Can you work these out from the drawing? Everything is in mm from the part's minimum corner. A direction names the side the tool comes from. Round coordinates to 2 decimals unless told otherwise and drop trailing zeros. Write each loop counter-clockwise with the first axis right and the second up, starting at its lowest first coordinate (ties: lowest second). Pieces come first, ordered by that corner, then holes. Notation, with made-up numbers: (-11, 57.5) - (11, 57.5) arc R16 cw to (11, 80.5) - close; hole circle Ø10 at (9.5, 51.25). An arc over 180 degrees is marked (long way). One line per item, written item: value. Start each with the question number.
(1) If I drill on L1, parallel to X at y = 1.55, z = 4.25; L2, parallel to Z at x = 0.65, y = 2.2; L3, parallel to Z at x = 2.4, y = 1.5, over which ranges is the centre line in solid material (lowest first)? Write a range as from..to.
(2) I'm going to push flat-ended pins straight in: pin 1 Ø1 at (x, z) = (0.5, 12) entering from -Y; pin 2 Ø1 at (y, z) = (2, 2) entering from -X. Where does each tip first touch, or does it pass through?
(3) I want a section at D-D on z = 12.75. List the corners of the cut face in (x, y) for me.
(4) I want a section at C-C on z = 3.75. List the corners of the cut face in (x, y) for me, plus the area to 3 significant figures.
(5) I want a section at B-B on y = 1.5. List the corners of the cut face in (x, z) for me, plus the area to 3 significant figures.
(6) On a 3-axis mill with a long thin cutter (end or side, diameter ignored), from which of +Z, -Z, +X, -X, +Y, -Y can I reach the whole of each face in a straight line? I mean the marked faces 1 and 2. Say none if no direction works.
(7) I want a section at A-A on x = 1.75. List the corners of the cut face in (y, z) for me, plus the area to 3 significant figures.
(8) Thinking about a two-plate mould opening in Z: for the marked faces 3 and 4, which applies, +Z half, -Z half, draft (parallel to the pull), parting line (faces both ways), or undercut?
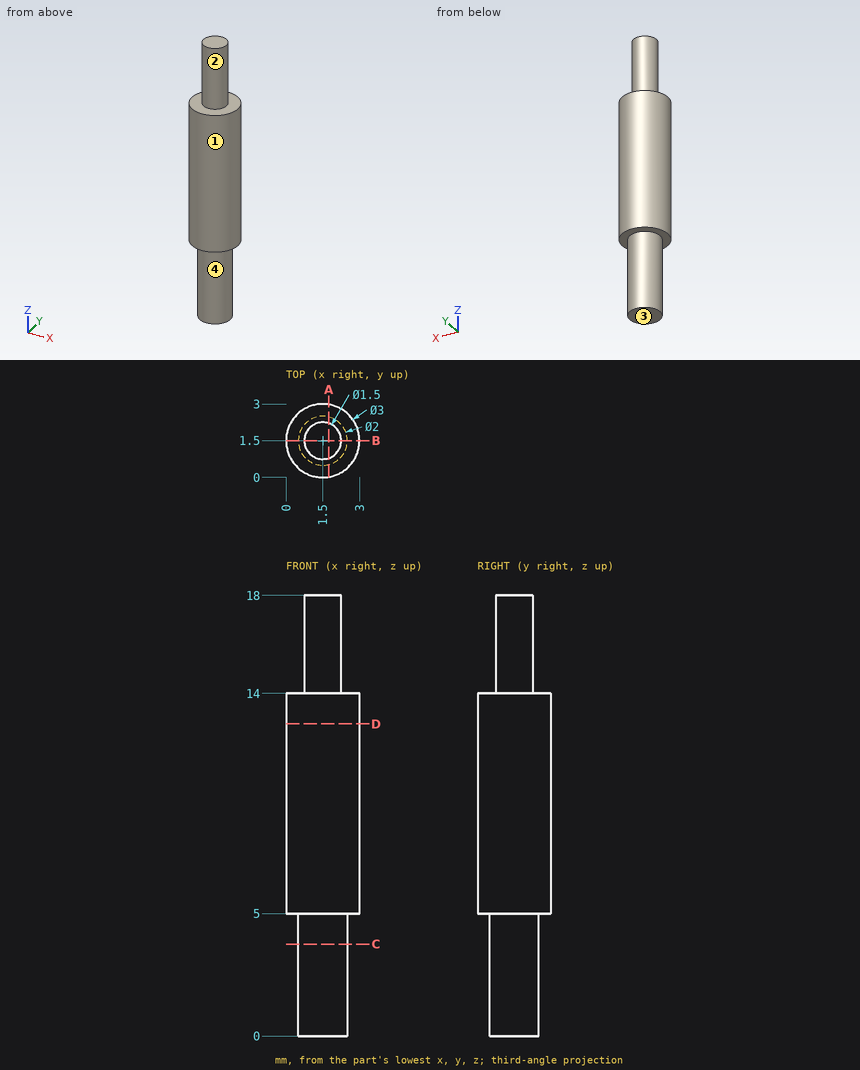
Established:
1. L1: 0.5..2.5
1. L2: 5..14
1. L3: 0..14
2. pin 1: y = 0.09
2. pin 2: x = 0.5
3. outline: circle Ø3 at (1.5, 1.5)
4. outline: circle Ø2 at (1.5, 1.5)
4. area: 3.14 mm2
5. outline: (0, 5) - (0.5, 5) - (0.5, 0) - (2.5, 0) - (2.5, 5) - (3, 5) - (3, 14) - (2.25, 14) - (2.25, 18) - (0.75, 18) - (0.75, 14) - (0, 14) - close
5. area: 43.0 mm2
6. face 1: +Z, -Z
6. face 2: +Z
7. outline: (0.02, 5) - (0.53, 5) - (0.53, 0) - (2.47, 0) - (2.47, 5) - (2.98, 5) - (2.98, 14) - (2.21, 14) - (2.21, 18) - (0.79, 18) - (0.79, 14) - (0.02, 14) - close
7. area: 42.0 mm2
8. face 3: -Z half
8. face 4: draft
